Check sheet for the drawn part. Datum: minimum x, y, z corner. Units: mm. Give positions to 0.01 mm unless a question says otherwise; leave off trailing zeros.
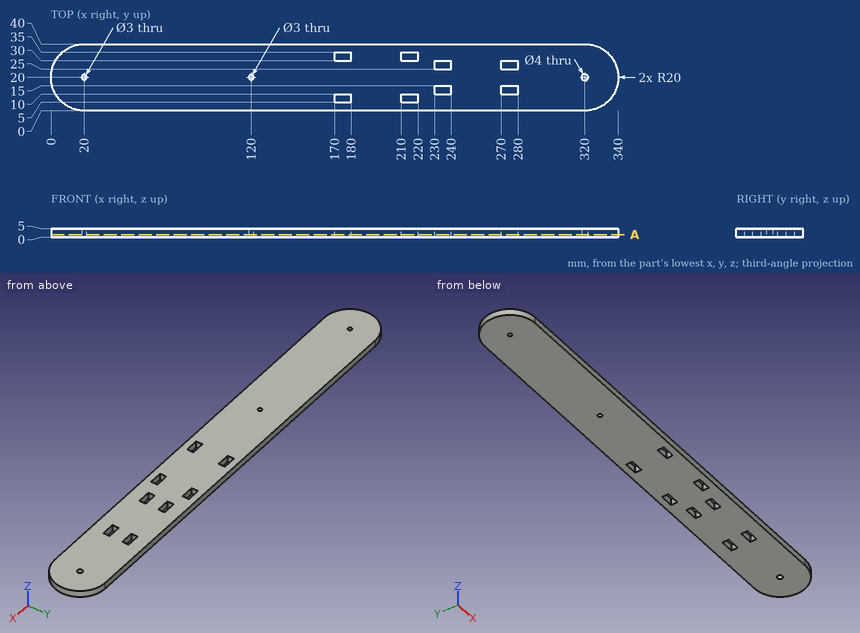
(1) Section check A-A, the plane z = 1.5. Give the number of separate pieces and of enclosed holes in the cut face, then the cut area to 3 significant figures.
Solved:
separate pieces: 1
enclosed holes: 11
area: 12,800 mm2
(2) Go/stop test with flat-tipped pins: pin 1 (1.5 mm diameter, centred on x = 217.5, z = 2, fed in from -Y); pin 2 (1.5 mm diameter, centred on y = 8, z = 2, fed in from -X); pin 3 (2.5 mm diameter, centred on y = 13, z = 2, fed in from +X); pin 4 (1 mm diameter, centred on y = 20, z = 3, fed in from +X). Record where each tip stops, or that it passes through.
Solved:
pin 1: stops at y = 0
pin 2: stops at x = 3.46
pin 3: stops at x = 339.16
pin 4: stops at x = 340
(3) Scan lines: line 1 (Y direction, x = 279, z = 1.95); line 2 (Y direction, x = 20, z = 1.7); line 3 (X direction, y = 11.5, z = 0.25). Record each from-to range of solid material in increasing order.
Solved:
line 1: y = 0 to 10, 15 to 25, 30 to 40
line 2: y = 0 to 18.5, 21.5 to 40
line 3: x = 1.9 to 230, 240 to 270, 280 to 338.1
